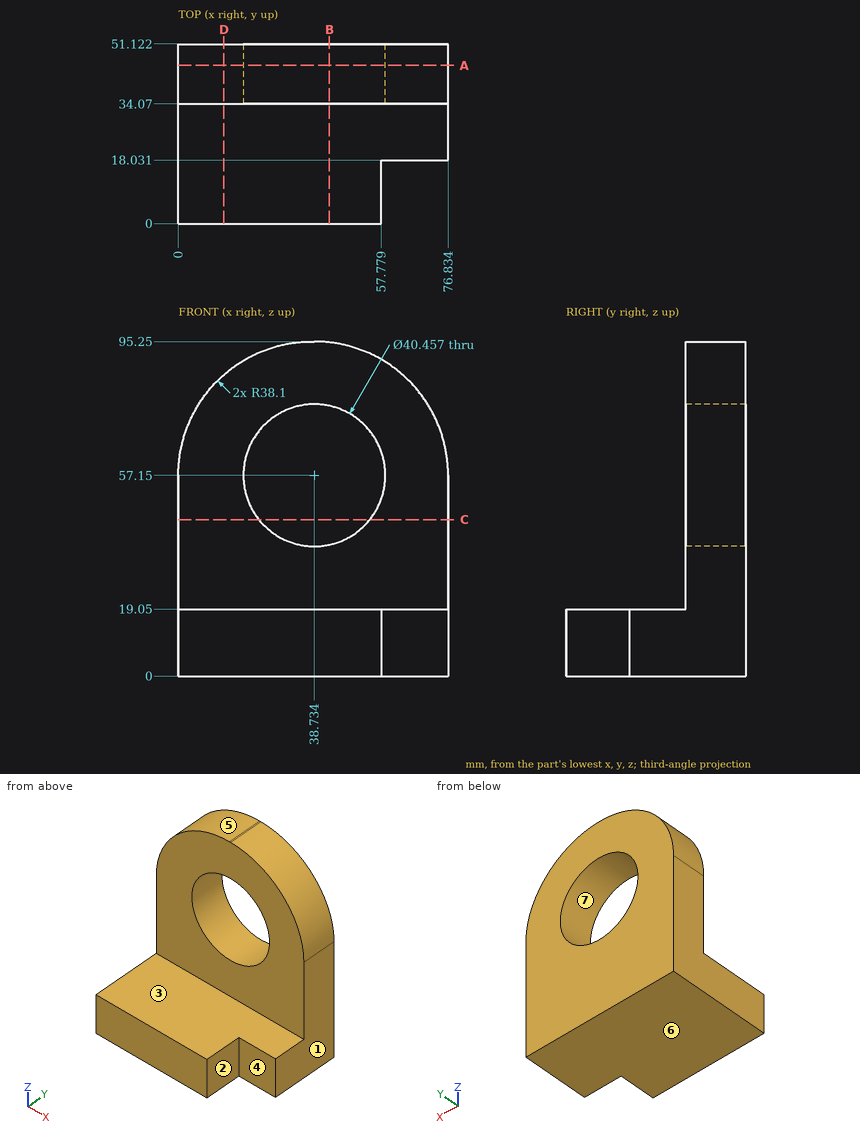
Check sheet for the drawn part. Datum: minimum x, y, z corner. Units: mm. A direction names the side the tool comes from. Give positions to 0.01 mm unless a question says otherwise; leave off trailing zeros. Loops run counter-clockwise (first coordinate to the right, second up) from the corner with the lowest first, then second, coordinate; pieces in that order, holes last.
1) Draft check along Z on the marked faces 4, 5, 6 and 7. Enter one of: pulls with the +Z half, pulls with the -Z half, needs draft (parallel to the pull), parting line crosses it, or undercut.
2) Depth check by flat-ended pin: pin 1 Ø23 at (x, z) = (40, 73) entering from -Y; pin 2 Ø8 at (x, y) = (28, 24) entering from -Z; pin 3 Ø9 at (y, z) = (11, 8.5) entering from +X; pin 4 Ø5.5 at (x, z) = (70.5, 7) entering from -Y. Enter the tip coordinate at first touch or a pass-through.
3) Sectioned sample at A-A, the plane y = 45. Enter the section's corners in (x, z), then the cut area to 3 significant figures.
4) Set-up check for the marked faces 1, 2 and 3: record each of +Z, -Z, +X, -X, +Y, -Y from which the full face is reachable in a straight line by a thin tool's end or side.
5) Sectioned sample at C-C, the plane z = 44.5. Enter the section's corners in (x, y), then the cut area to 3 significant figures.
6) Sectioned sample at D-D, the plane x = 13. Enter the section's corners in (y, z).
7) Thickness scan on line 1 along Y through (x, z) = (25.5, 20.5); line 2 along X through (y, z) = (47, 57) (1 decimal); line 3 along Z through (x, y) = (57, 27.5). Record the ranges inside material, lowest first.
8) Sectioned sample at B-B, the plane x = 43. Enter the section's corners in (y, z).
Answers:
1. face 4: needs draft
1. face 5: pulls with the +Z half
1. face 6: pulls with the -Z half
1. face 7: undercut
2. pin 1: stops at y = 34.07
2. pin 2: stops at z = 0
2. pin 3: stops at x = 57.78
2. pin 4: stops at y = 18.03
3. outline: (0, 0) - (76.83, 0) - (76.83, 57.15) arc R38.1 ccw to (38.73, 95.25) - (38.1, 95.25) arc R38.1 ccw to (0, 57.15) - close; hole circle Ø40.46 at (38.73, 57.15)
3. area: 5,410 mm2
4. face 1: +Z, -Z, +X, +Y, -Y
4. face 2: +Z, -Z, +X, -Y
4. face 3: +Z, +X, -X, -Y
5. outline: (0, 34.07) - (22.95, 34.07) - (22.95, 51.12) - (0, 51.12) - close; (54.52, 34.07) - (76.83, 34.07) - (76.83, 51.12) - (54.52, 51.12) - close
5. area: 772 mm2
6. outline: (0, 0) - (51.12, 0) - (51.12, 85.81) - (34.07, 85.81) - (34.07, 19.05) - (0, 19.05) - close
7. line 1: y = 34.07 to 51.12
7. line 2: x = 0 to 18.5, 59 to 76.8
7. line 3: z = 0 to 19.05
8. outline: (0, 0) - (51.12, 0) - (51.12, 37.38) - (34.07, 37.38) - (34.07, 19.05) - (0, 19.05) - close; (34.07, 76.92) - (51.12, 76.92) - (51.12, 95.01) - (34.07, 95.01) - close
